Here's how the part is built. I have some questions about the finished solid (model axes, mm). Face numbers are marked on the shaded views. A direction names the side the tool comes from. Coordinates: 2 decimals unless noted, no trailing zeros. Answer in a Markdown table with one row per item. Add a question column.
Item 1: Imagine slicing it at A-A (y = -23.5). State how many separate pieces and enclosed holes the cut face has, plus the area to 3 significant figures.
Item 2: We'd pull the mould along X, two halves only. Please class the marked faces 1, 2 and 3: +X half, -X half, draft (parallel to the pull), parting line (faces both ways), or undercut.
Item 3: Which directions (+Z, -Z, +X, -X, +Y, -Y) give clear straight access to the entire face, cutting with the end or side of a thin tool? Please do the marked faces 4 and 5.
Item 4: If I drill on probe 1 along X at (y, z) = (-19.5, 2); probe 2 along Y at (x, z) = (7, 3.5); probe 3 along Y at (x, z) = (21.5, 4), over which ranges is the centre line in solid material (lowest first)? Write a range as from..to.
Item 5: I'm going to push flat-ended pins straight in: pin 1 (1.5 mm diameter, centred on x = -17, z = 4, fed in from +Y); pin 2 (10 mm diameter, centred on x = 0, y = -13.83, fed in from -Z); pin 3 (3 mm diameter, centred on y = 19, z = 1, fed in from -X); pin 4 (10 mm diameter, centred on x = 0, y = -26.12, fed in from +Z). Where does each tip first touch, or does it pass through?
from build123d import *

# Parameters (mm, degrees)
F3_DEPTH = 2.54
F4_R     = 6.006136
F4_R_2   = 4.291362
F4_R_3   = 3.841772
F5_DEPTH = 25.4
F7_DEPTH = 3.81
F8_R     = 1.651
F9_DEPTH = 25.4


with BuildPart() as f1:
    # F0 (on Front) → F1 (revolve)
    with BuildSketch(Plane.XZ):
        with BuildLine():
            Line((0, 4.572), (0, 0))
            Line((0, 0), (31.75, 0))
            ThreePointArc((31.75, 0), (30.718062, 2.286), (31.75, 4.572))
            Line((31.75, 4.572), (0, 4.572))
        make_face()
    revolve(axis=Axis((0, 0, 2.286), (0, 0, 1)))

    # F2 (on face) → F3 (join)
    with BuildSketch(Plane.XY.offset(4.572)):
        Polygon((-0.058218, 8.798626), (-7.648942, 4.348895), (-7.590724, -4.449731), (0.058218, -8.798626), (7.648942, -4.348895), (7.590724, 4.449731), align=None)
    extrude(amount=F3_DEPTH)

    # F4 (on face) → F5 (cut)
    with BuildSketch(Plane.XY.offset(4.572)):
        with Locations((-11.983808, 20.4447)):
            Circle(F4_R)
        with Locations((0, 13.830239)):
            Circle(F4_R_2)
        with Locations((0, 26.124066)):
            Circle(F4_R_3)
        with Locations((11.713726, 20.600633)):
            Circle(F4_R)
        with Locations((11.977333, 6.915986)):
            Circle(F4_R_2)
        with Locations((23.697534, 0.155932)):
            Circle(F4_R)
        with Locations((22.624847, -13.060728)):
            Circle(F4_R_3)
        with Locations((11.97808, -6.913814)):
            Circle(F4_R_2)
        with Locations((11.983808, -20.4447)):
            Circle(F4_R)
        with Locations((0.001496, -26.123189)):
            Circle(F4_R_3)
        with Locations((0.001496, -13.829362)):
            Circle(F4_R_2)
        with Locations((-11.713726, -20.600633)):
            Circle(F4_R)
        with Locations((-11.975837, -6.91511)):
            Circle(F4_R_2)
        with Locations((-23.697534, -0.155932)):
            Circle(F4_R)
        with Locations((-22.623351, 13.061604)):
            Circle(F4_R_3)
        with Locations((-11.976585, 6.914691)):
            Circle(F4_R_2)
        with Locations((-22.622603, -13.062023)):
            Circle(F4_R_3)
        with Locations((22.624099, 13.0629)):
            Circle(F4_R_3)
    extrude(amount=-F5_DEPTH, mode=Mode.SUBTRACT)

    # F6 (on face) → F7 (cut)
    with BuildSketch(Plane.XY.offset(7.112)):
        Polygon((6.300916, 3.604427), (0.028933, 7.258967), (-6.271984, 3.65454), (-6.300916, -3.604427), (-0.028933, -7.258967), (6.271984, -3.65454), align=None)
    extrude(amount=-F7_DEPTH, mode=Mode.SUBTRACT)

    # F8 (on face) → F9 (cut)
    with BuildSketch(Plane.XY.offset(3.302)):
        Circle(F8_R)
    extrude(amount=-F9_DEPTH, mode=Mode.SUBTRACT)


solid = f1.part
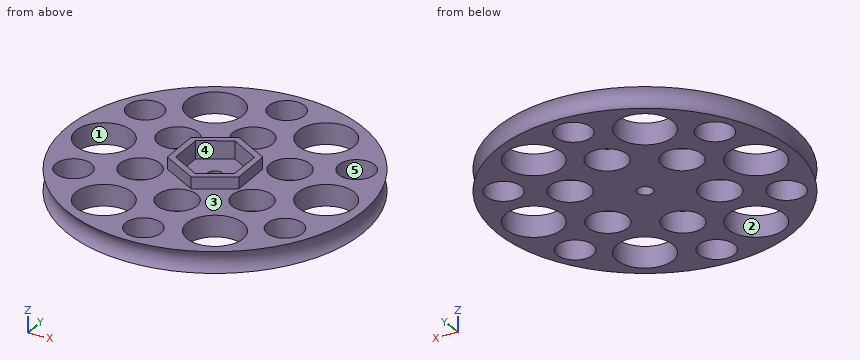
Here are the results:
| question | item | result |
|---|---|---|
| 1 | separate pieces | 4 |
| 1 | enclosed holes | 0 |
| 1 | area | 64.3 mm2 |
| 2 | face 1 | undercut |
| 2 | face 2 | undercut |
| 2 | face 3 | draft |
| 3 | face 4 | +Z |
| 3 | face 5 | +Z, -Z |
| 4 | probe 1 | x = -23.75..-17.62, -5.81..6.05, 17.92..23.75 |
| 4 | probe 2 | y = -30.17..-23.8, -17.09..16.88, 24.32..30.17 |
| 4 | probe 3 | y = -22.67..-16.73, -9.39..-5.43, 5.75..9.39, 16.74..22.67 |
| 5 | pin 1 | stops at y = 27.12 |
| 5 | pin 2 | stops at z = 0 |
| 5 | pin 3 | stops at x = -26.24 |
| 5 | pin 4 | stops at z = 4.57 |
